Build history of the part. All positions in model axes, mm. Face numbers are marked on the shaded views. A direction names the side the tool comes from. Give positions to 0.01 mm unless a question says otherwise; leave off trailing zeros. Write each loop counter-clockwise with the first axis right and the second up, starting at its lowest first coordinate (ties: lowest second). Pieces come first, ordered by that corner, then holes. Notation, with made-up numbers: M 70,71.25 L 118,71.25 A24 ccw 118,106.25 Z; hole C -26,74 d10. An arc over 180 degrees is marked long. One line per item, written item: value. Start each with the question number.
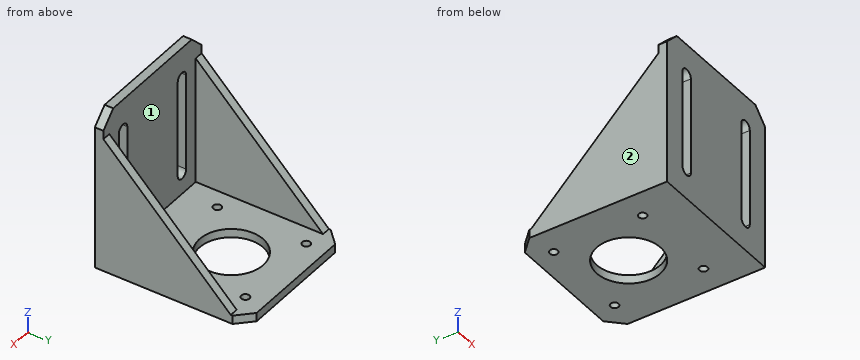
from build123d import *

# Parameters (mm, degrees)
CROQUIS1_R              = 11.1
SALIENTE_EXTRUIR2_DEPTH = 3
CROQUIS2_R              = 1.4
CORTAR_EXTRUIR1_DEPTH   = 40.550600501
CROQUIS3_W              = 50
CROQUIS3_H              = 3
SALIENTE_EXTRUIR3_DEPTH = 52.4
CORTAR_EXTRUIR2_DEPTH   = 81.64217259
SALIENTE_EXTRUIR4_DEPTH = 3


with BuildPart() as part:
    # Croquis1 → Saliente-Extruir2 (new body)
    with BuildSketch(Plane.XY):
        Polygon((20, 22.5), (-20, 22.5), (-25, 17.5), (-25, -30.5), (25, -30.5), (25, 17.5), align=None)
        Circle(CROQUIS1_R, mode=Mode.SUBTRACT)
    extrude(amount=SALIENTE_EXTRUIR2_DEPTH)

    # Croquis2 → Cortar-Extruir1 (cut, through all)
    with BuildSketch(Plane.XY.offset(3)):
        with Locations((-15.5, 15.5)):
            Circle(CROQUIS2_R)
        with Locations((15.5, 15.5)):
            Circle(CROQUIS2_R)
        with Locations((15.5, -15.5)):
            Circle(CROQUIS2_R)
        with Locations((-15.5, -15.5)):
            Circle(CROQUIS2_R)
    extrude(amount=-CORTAR_EXTRUIR1_DEPTH, mode=Mode.SUBTRACT)

    # Croquis3 → Saliente-Extruir3 (add)
    with BuildSketch(Plane.XY.offset(3)):
        with Locations((0, -29)):
            Rectangle(CROQUIS3_W, CROQUIS3_H)
    extrude(amount=SALIENTE_EXTRUIR3_DEPTH)

    # Croquis4 → Cortar-Extruir2 (cut, through all)
    with BuildSketch(Plane.XZ.offset(30.5)):
        Polygon((-25, 50.4), (-20, 55.4), (-25, 55.4), align=None)
        with BuildLine():
            Line((-17.15, 44.4), (-17.15, 10.6))
            ThreePointArc((-17.15, 10.6), (-15, 8.45), (-12.85, 10.6))
            Line((-12.85, 10.6), (-12.85, 44.4))
            ThreePointArc((-12.85, 44.4), (-15, 46.55), (-17.15, 44.4))
        make_face()
        with BuildLine():
            Line((12.85, 44.4), (12.85, 10.6))
            ThreePointArc((12.85, 10.6), (15, 8.45), (17.15, 10.6))
            Line((17.15, 10.6), (17.15, 44.4))
            ThreePointArc((17.15, 44.4), (15, 46.55), (12.85, 44.4))
        make_face()
        Polygon((25, 55.4), (25, 50.4), (20, 55.4), align=None)
    extrude(amount=-CORTAR_EXTRUIR2_DEPTH, mode=Mode.SUBTRACT)

    # Croquis5 → Saliente-Extruir4 (add)
    with BuildSketch(Plane.ZY.offset(25)):
        Polygon((3, 16.9), (3, -27.5), (47.4, -27.5), align=None)
    saliente_extruir4 = extrude(amount=-SALIENTE_EXTRUIR4_DEPTH)

    # Simetría1: Saliente-Extruir4 across plane
    add(saliente_extruir4.mirror(Plane(origin=(0, 0, 0), x_dir=(0, 0, 1), z_dir=(1, 0, 0))))


solid = part.part
1) Band-saw the part on D-D (z = 4). List the corners of the cut face in (x, y), then the cut area to 3 significant figures.
2) Tool access for the marked faces 1 and 2: list every direction of +Z, -Z, +X, -X, +Y, -Y with a clear straight run to the whole face (end or side of a thin tool).
3) Probe line 1 along Y through (x, z) = (-15.5, 1.75); line 2 along X through (y, z) = (-28, 31); line 3 along X through (y, z) = (15, 2). List the from-to ranges inside material, lowest first. Write a range as from..to.
4) Band-saw the part on C-C (x = 15). List the corners of the cut face in (y, z).
5) Band-saw the part on A-A (z = 23). List the corners of the cut face in (x, y), then the cut area to 3 significant figures.
6) Drop a flat-ended pin along its axis: P1, Ø3, axis at x = 12, y = 15.5, coming from the +Z side. Give the stop position or say it passes through.
7) Band-saw the part on B-B (y = 0). List the corners of the cut face in (x, z).
Model answer:
1. outline: M -25,-30.5 L 25,-30.5 L 25,15.9 L 22,15.9 L 22,-27.5 L -22,-27.5 L -22,15.9 L -25,15.9 Z
1. area: 410 mm²
2. face 1: +Z, +Y
2. face 2: +Z, -Z, -X, +Y, -Y
3. line 1: y = -30.5..-16.9, -14.1..14.1, 16.9..22.5
3. line 2: x = -25..-17.15, -12.85..12.85, 17.15..25
3. line 3: x = -25..-16.81, -14.19..14.19, 16.81..25
4. outline: M -30.5,0 L -16.81,0 L -16.81,3 L -27.5,3 L -27.5,8.45 L -30.5,8.45 Z; M -30.5,46.55 L -27.5,46.55 L -27.5,55.4 L -30.5,55.4 Z; M -14.19,0 L 14.19,0 L 14.19,3 L -14.19,3 Z; M 16.81,0 L 22.5,0 L 22.5,3 L 16.81,3 Z
5. outline: M -25,-30.5 L -17.15,-30.5 L -17.15,-27.5 L -22,-27.5 L -22,-3.1 L -25,-3.1 Z; M -12.85,-30.5 L 12.85,-30.5 L 12.85,-27.5 L -12.85,-27.5 Z; M 17.15,-30.5 L 25,-30.5 L 25,-3.1 L 22,-3.1 L 22,-27.5 L 17.15,-27.5 Z
5. area: 271 mm²
6. P1: stops at z = 3
7. outline: M -25,0 L -11.1,0 L -11.1,3 L -22,3 L -22,19.9 L -25,19.9 Z; M 11.1,0 L 25,0 L 25,19.9 L 22,19.9 L 22,3 L 11.1,3 Z
